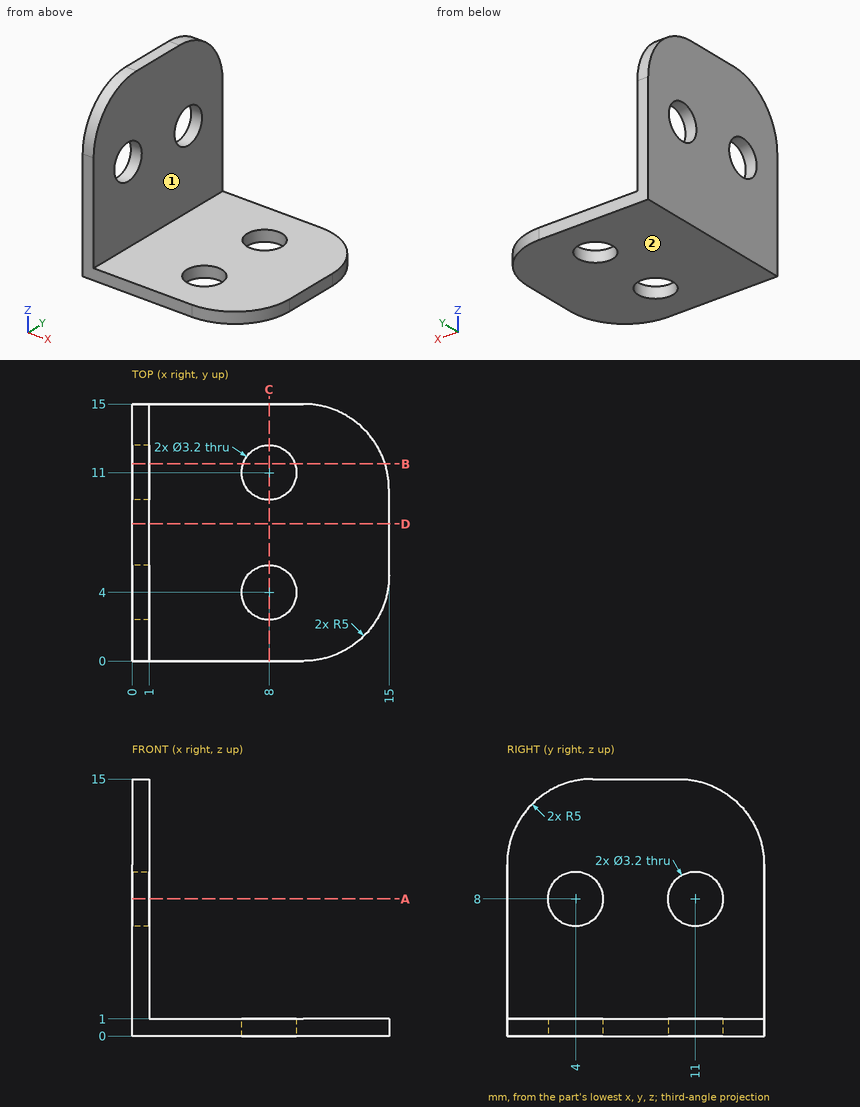
Check sheet for the drawn part. Datum: minimum x, y, z corner. Units: mm. A direction names the side the tool comes from. Round coordinates to 2 decimals unless told otherwise and drop trailing zeros. Order: outer loops, then holes, each group sorted by start corner. A loop starts at its lowest first (then second) coordinate and runs counter-clockwise, first axis right, second up.
(1) Cross-section at A-A, the plane z = 8. Enter the section's corners in (x, y).
(2) Scan lines: probe 1 along Y at (x, z) = (8, 0.35); probe 2 along Z at (x, y) = (1.75, 8.25). Record each from-to range of solid material in increasing order.
(3) Go/stop test with flat-tipped pins: P1, Ø3.5, axis at y = 4, z = 8, coming from the -X side; P2, Ø2, axis at y = 10, z = 2.5, coming from the +X side; P3, Ø7, axis at x = 8, y = 7, coming from the +Z side. Record where each tip stops, or that it passes through.
(4) Cross-section at D-D, the plane y = 8. Enter the section's corners in (x, z), and give its area (3 significant figures).
(5) Cross-section at C-C, the plane x = 8. Enter the section's corners in (y, z).
(6) Cross-section at B-B, the plane y = 11.5. Enter the section's corners in (x, z), and give its area (3 significant figures).
(7) Access from +Z, -Z, +X, -X, +Y, -Y to the whole of each face (thin tool, end or side, straight path). Record for the marked faces 1 and 2.
Check sheet entries:
1. outline: (0, 0) - (1, 0) - (1, 2.4) - (0, 2.4) - close; (0, 5.6) - (1, 5.6) - (1, 9.4) - (0, 9.4) - close; (0, 12.6) - (1, 12.6) - (1, 15) - (0, 15) - close
2. probe 1: y = 0 to 2.4, 5.6 to 9.4, 12.6 to 15
2. probe 2: z = 0 to 1
3. P1: stops at x = 0
3. P2: stops at x = 1
3. P3: stops at z = 1
4. outline: (0, 0) - (15, 0) - (15, 1) - (1, 1) - (1, 15) - (0, 15) - close
4. area: 29.0 mm2
5. outline: (0, 0) - (2.4, 0) - (2.4, 1) - (0, 1) - close; (5.6, 0) - (9.4, 0) - (9.4, 1) - (5.6, 1) - close; (12.6, 0) - (15, 0) - (15, 1) - (12.6, 1) - close
6. outline: (0, 0) - (6.48, 0) - (6.48, 1) - (1, 1) - (1, 6.48) - (0, 6.48) - close; (0, 9.52) - (1, 9.52) - (1, 14.77) - (0, 14.77) - close; (9.52, 0) - (14.77, 0) - (14.77, 1) - (9.52, 1) - close
6. area: 22.5 mm2
7. face 1: +Z, +X, +Y, -Y
7. face 2: -Z, +X, -X, +Y, -Y
